Build history of the part. All positions in model axes, mm. Coordinates: 2 decimals unless noted, no trailing zeros. Order: outer loops, then holes, each group sorted by start corner. A loop starts at its lowest first (then second) coordinate and runs counter-clockwise, first axis right, second up. Notation, with made-up numbers: (-21, 18) - (4, 18) arc R10 ccw to (4, 34) - close; hole circle Ø10 at (73, -38.5). An arc over 180 degrees is marked (long way). Write each question's results on one line, items separated by ' | '.
from build123d import *

# Parameters (mm, degrees)
F0_W     = 266
F0_H     = 172
F1_DEPTH = 3.2
F2_R     = 5
F3_R     = 2
F4_R     = 2.3534685549
F5_DEPTH = 0.1


with BuildPart() as f1:
    # F0 (on Front) → F1 (new body, symmetric)
    with BuildSketch(Plane.XZ):
        with Locations((7.3433928192, 9.1417450992)):
            Rectangle(F0_W, F0_H)
    extrude(amount=F1_DEPTH, both=True)

    # F2
    f2_edges = [f1.edges().sort_by_distance(p)[0] for p in [
        (-125.656607, 0, 95.141745),
        (140.343393, 0, 95.141745),
        (140.343393, 0, -76.858255),
        (-125.656607, 0, -76.858255),
    ]]
    fillet(f2_edges, radius=F2_R)

    # F3
    f3_edges = [f1.edges().sort_by_distance(p)[0] for p in [
        (7.343393, 3.2, -76.858255),
        (7.343393, -3.2, -76.858255),
        (-125.656607, 3.2, 9.141745),
        (-125.656607, -3.2, 9.141745),
        (7.343393, 3.2, 95.141745),
        (140.343393, 3.2, 9.141745),
        (140.343393, -3.2, 9.141745),
        (7.343393, -3.2, 95.141745),
        (-124.192141, -3.2, -75.393789),
        (-124.192141, 3.2, -75.393789),
        (-124.192141, -3.2, 93.677279),
        (-124.192141, 3.2, 93.677279),
        (138.878927, -3.2, 93.677279),
        (138.878927, 3.2, -75.393789),
        (138.878927, -3.2, -75.393789),
        (138.878927, 3.2, 93.677279),
    ]]
    fillet(f3_edges, radius=F3_R)

    # F4 (on face) → F5 (join)
    with BuildSketch(Plane(origin=(0, 3.2, 0), x_dir=(-1, 0, 0), z_dir=(0, 1, 0))):
        with Locations((117.853499949, 87.8090560436)):
            Circle(F4_R)
    extrude(amount=F5_DEPTH)


solid = f1.part
1. Drop a flat-ended pin along its axis: pin 1 Ø6 at (x, z) = (-52.5, 26) entering from +Y. Give the stop position or say it passes through.
Solved:
pin 1: stops at y = 3.2
2. Band-saw the part on B-B on x = -48.5. Give the cut face in (y, z), then the cut area to 3 significant figures.
Solved:
outline: (-3.2, -74.86) arc R2 ccw to (-1.2, -76.86) - (1.2, -76.86) arc R2 ccw to (3.2, -74.86) - (3.2, 93.14) arc R2 ccw to (1.2, 95.14) - (-1.2, 95.14) arc R2 ccw to (-3.2, 93.14) - close | area: 1,100 mm2
3. Band-saw the part on A-A on z = -62. Give the cut face in (x, y).
Solved:
outline: (-125.66, -1.2) arc R2 ccw to (-123.66, -3.2) - (138.34, -3.2) arc R2 ccw to (140.34, -1.2) - (140.34, 1.2) arc R2 ccw to (138.34, 3.2) - (-123.66, 3.2) arc R2 ccw to (-125.66, 1.2) - close
4. Probe line 1 (Y direction, x = 8, z = 21.5); line 2 (Z direction, x = -75.5, y = -1.5); line 3 (X direction, y = 2.25, z = -13). List the from-to ranges inside material, lowest first.
Solved:
line 1: y = -3.2 to 3.2 | line 2: z = -76.84 to 95.12 | line 3: x = -125.36 to 140.05
